Here's how the part is built. I have some questions about the finished solid (model axes, mm). Face numbers are marked on the shaded views. Give positions to 0.01 mm unless a question says otherwise; leave off trailing zeros. Loops run counter-clockwise (first coordinate to the right, second up) from the corner with the lowest first, then second, coordinate; pieces in that order, holes last.
Q1. If we section it at D-D (z = 6): Please give me the cut outline in (x, y).
Q2. If we section it at A-A (x = 0): Please give me the cut outline in (y, z), plus the area to 3 significant figures.
Q3. Will these pins go through, and if not, where does the flat tip stop? P1, Ø10, axis at x = 8, y = 5.5, coming from the -Z side; P2, Ø2, axis at y = 10, z = 5, coming from the -X side; P3, Ø4, axis at y = -10, z = 8.5, coming from the +X side.
Q4. We'd pull the mould along X, two halves only. Please class the marked faces 1, 2, 3 and 4: +X half, -X half, draft (parallel to the pull), parting line (faces both ways), or undercut.
Q5. If we section it at C-C (y = -10.5): Please give me the cut outline in (x, z), plus the area to 3 significant figures.
Q6. I need wall thicknesses on line 1 (Y direction, x = 0, z = 3.5); line 2 (X direction, y = 11.5, z = 2.75); line 3 (X direction, y = 13, z = 5.5). Which ranges of each line are inside material? Lowest first, please.
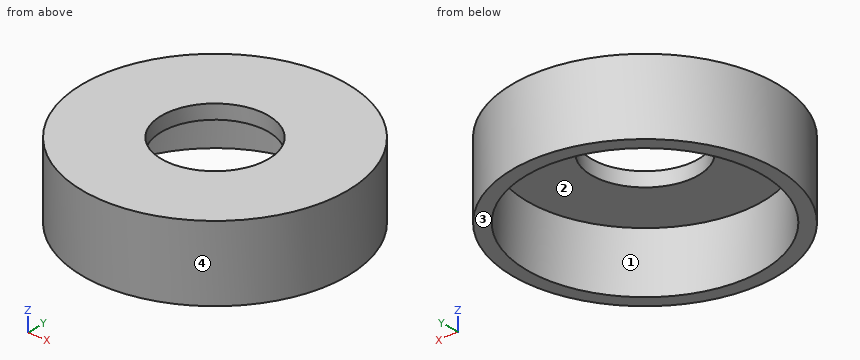
from build123d import *

# Parameters (mm, degrees)
F0_R     = 18.5
F1_DEPTH = 10.5
F2_T     = -2
F3_R     = 7.5
F4_DEPTH = 2


with BuildPart() as f1:
    # F0 (on Top) → F1 (new body)
    with BuildSketch(Plane.XY):
        Circle(F0_R)
    extrude(amount=F1_DEPTH)

    # F2
    f2_openings = [f1.faces().sort_by_distance(p)[0] for p in [
        (0, 0, 0),
    ]]
    offset(amount=F2_T, openings=f2_openings)

    # F3 (on face) → F4 (cut, through all)
    with BuildSketch(Plane.XY.offset(10.5)):
        Circle(F3_R)
    extrude(amount=-F4_DEPTH, mode=Mode.SUBTRACT)


solid = f1.part
Check sheet entries:
1. outline: circle Ø37 at (0, 0); hole circle Ø33 at (0, 0)
2. outline: (-18.5, 0) - (-16.5, 0) - (-16.5, 8.5) - (-7.5, 8.5) - (-7.5, 10.5) - (-18.5, 10.5) - close; (7.5, 8.5) - (16.5, 8.5) - (16.5, 0) - (18.5, 0) - (18.5, 10.5) - (7.5, 10.5) - close
2. area: 78.0 mm2
3. P1: stops at z = 8.5
3. P2: stops at x = -16.16
3. P3: stops at x = 16.68
4. face 1: undercut
4. face 2: undercut
4. face 3: draft
4. face 4: parting line
5. outline: (-15.23, 0) - (-12.73, 0) - (-12.73, 8.5) - (12.73, 8.5) - (12.73, 0) - (15.23, 0) - (15.23, 10.5) - (-15.23, 10.5) - close
5. area: 103 mm2
6. line 1: y = -18.5 to -16.5, 16.5 to 18.5
6. line 2: x = -14.49 to -11.83, 11.83 to 14.49
6. line 3: x = -13.16 to -10.16, 10.16 to 13.16
